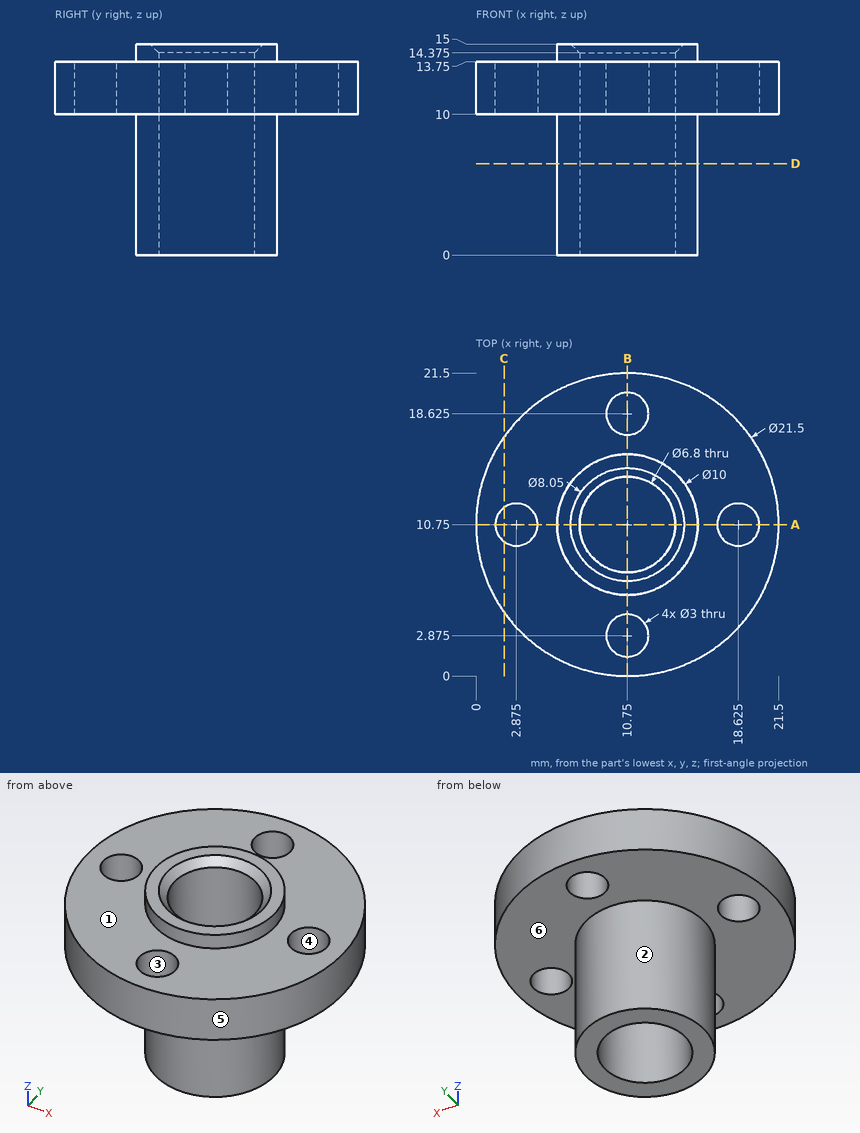
Source: three-view drawing plus pictorial views. Frame: mm from the lowest corner of the part. A direction names the side the tool comes from. Give positions to 0.01 mm unless a question says otherwise; leave off trailing zeros. Loops run counter-clockwise (first coordinate to the right, second up) from the corner with the lowest first, then second, coordinate; pieces in that order, holes last. Notation, with made-up numbers: (60.25, -12) -> (90.25, -12) arc R7 cw to (90.25, -5) -> close; hole circle Ø6 at (-11, -18.75). An arc over 180 degrees is marked (long way). Use a Markdown table: item, result. Add a question column.
(1) Section query A-A (y = 10.75). Output: boundary loops of the cut face in (x, z) (3 decimals), then the cut area to 3 significant figures.
(2) Pull-direction query (Y, two-part tool) for the marked faces 4, 5 and 6; classes: +Y half, -Y half, draft (parallel to the pull), parting line (faces both ways), or undercut.
(3) Ray query, line 1 (Y direction, x = 10.75, z = 11.15) (3 decimals); line 2 (Z direction, x = 10.75, y = 17); line 3 (Y direction, x = 8.25, z = 4.25). Return the intervals inside material, ascending.
(4) Access query for the marked faces 1, 2 and 3. Directions: +Z, -Z, +X, -X, +Y, -Y. A direction counts if a zero-diameter tool reaches every point of the face in a straight line with its end or side. Return the directions, or none.
(5) First-contact query: pin 1 Ø3 at (x, y) = (18.5, 15.5) entering from -Z; pin 2 Ø6.5 at (x, y) = (15, 14) entering from +Z; pin 3 Ø5 at (x, z) = (17, 9) entering from +Y; pin 4 Ø1.5 at (y, z) = (13.5, 8) entering from -X. Flat tips, straight axial feed; report the tip coordinate or a pass-through.
(6) Section query D-D (z = 6.5). Output: boundary loops of the cut face in (x, y), then the cut area to 3 significant figures.
(7) Section query C-C (x = 2). Output: boundary loops of the cut face in (y, z) (3 decimals), then the cut area to 3 significant figures.
Checked values:
| question | item | result |
|---|---|---|
| 1 | outline | (0, 10) -> (1.375, 10) -> (1.375, 13.75) -> (0, 13.75) -> close; (4.375, 10) -> (5.75, 10) -> (5.75, 0) -> (7.35, 0) -> (7.35, 14.375) -> (6.725, 15) -> (5.75, 15) -> (5.75, 13.75) -> (4.375, 13.75) -> close; (14.15, 0) -> (15.75, 0) -> (15.75, 10) -> (17.125, 10) -> (17.125, 13.75) -> (15.75, 13.75) -> (15.75, 15) -> (14.775, 15) -> (14.15, 14.375) -> close; (20.125, 10) -> (21.5, 10) -> (21.5, 13.75) -> (20.125, 13.75) -> close |
| 1 | area | 68.2 mm^2 |
| 2 | face 4 | undercut |
| 2 | face 5 | parting line |
| 2 | face 6 | draft |
| 3 | line 1 | 0 to 1.375, 4.375 to 7.35, 14.15 to 17.125, 20.125 to 21.5 |
| 3 | line 2 | 10 to 13.75 |
| 3 | line 3 | 6.42 to 8.45, 13.05 to 15.08 |
| 4 | face 1 | +Z |
| 4 | face 2 | -Z |
| 4 | face 3 | +Z, -Z |
| 5 | pin 1 | z = 10 |
| 5 | pin 2 | z = 15 |
| 5 | pin 3 | y = 20.74 |
| 5 | pin 4 | x = 6.17 |
| 6 | outline | circle Ø10 at (10.75, 10.75); hole circle Ø6.8 at (10.75, 10.75) |
| 6 | area | 42.2 mm^2 |
| 7 | outline | (4.505, 10) -> (9.532, 10) -> (9.532, 13.75) -> (4.505, 13.75) -> close; (11.968, 10) -> (16.995, 10) -> (16.995, 13.75) -> (11.968, 13.75) -> close |
| 7 | area | 37.7 mm^2 |
